CAD build for the part. Positions are in the model's coordinates, mm. A direction names the side the tool comes from. Round coordinates to 2 decimals unless told otherwise and drop trailing zeros. Order: outer loops, then holes, each group sorted by start corner. A loop starts at its lowest first (then second) coordinate and runs counter-clockwise, first axis right, second up. Notation, with made-up numbers: (-21, 52.25) - (8, 52.25) arc R26 cw to (8, 69.25) - close; hole circle Ø10 at (74.25, -20). An arc over 180 degrees is marked (long way). Use one line per item in the form item = value. Start each with the question number.
Autodesk Inventor part; units mm, degrees
ref_plane "Work Plane1" through (443.7901, 0, 457.2) normal (-0.7071, 0, 0.7071) x (0, -1, 0)
ref_plane "YZ Plane" through (0, 0, 0) normal (1, 0, 0) x (0, 1, 0)
ref_plane "XZ Plane" through (0, 0, 0) normal (0, 1, 0) x (-1, 0, 0)
sketch "Sketch1" plane through (0, 0, 0) normal (0, 0, 1) x (1, 0, 0)
  line L0 (-13.4099, 13.8043) -> (443.7901, 13.8043)
  line L1 (443.7901, 13.8043) -> (443.7901, -443.3957)
  line L2 (443.7901, -443.3957) -> (-13.4099, -443.3957)
  line L3 (-13.4099, -443.3957) -> (-13.4099, 13.8043)
  point P0 (0, 0)
  dimension "d0" = 457.2
  dimension "d1" = 457.2
extrude "Extrusion1" add sketch "Sketch1" along normal blind 457.2
ref_plane "Work Plane1" through (443.7901, 0, 457.2) normal (-0.7071, 0, 0.7071) x (0, -1, 0)
sketch "Sketch2" plane through (0, 0, 457.2) normal (0, 0, 1) x (1, 0, 0)
  point P0 (0, 0)
sketch "Sketch3" plane through (0, 0, 457.2) normal (0, 0, 1) x (1, 0, 0)
  circle A0 centre (215.1901, -214.7957) radius 78.8174
  line L0 (443.7901, -443.3957) -> (443.7901, 13.8043)
  line L1 (443.7901, 13.8043) -> (-13.4099, 13.8043)
  point P0 (0, 0)
  dimension "d4" = 228.6
  dimension "d5" = 228.6
extrude "Extrusion2" add sketch "Sketch3" along normal blind 12.7
sketch "Sketch4" plane through (443.7901, -443.3957, 0) normal (1, 0, 0) x (0, 0, -1)
  point P0 (0, 443.3957)
sketch "Sketch5" plane through (443.7901, -443.3957, 0) normal (1, 0, 0) x (0, 0, -1)
  line L0 (0, 457.2) -> (-457.2, 0)
  circle A0 centre (-76.1993, 381.0007) radius 63.5
  circle A1 centre (-228.6, 228.6) radius 63.5
  circle A2 centre (-381.0007, 76.1993) radius 63.5
  point P0 (0, 443.3957)
  dimension "d21" = 127
  dimension "d22" = 127
  dimension "d23" = 127
  dimension "d25" = 646.5784
  dimension "d26" = 107.762
  dimension "d28" = 107.762
extrude "Extrusion3" add sketch "Sketch5" along normal blind 12.7
sketch "Sketch6" plane through (-13.4099, -443.3957, 0) normal (-1, 0, 0) x (0, 0, 1)
  line L0 (0, 457.2) -> (457.2, 0)
  line L1 (114.3, 342.9) -> (342.9, 342.9)
  line L2 (342.9, 342.9) -> (342.9, 114.3)
  line L3 (342.9, 114.3) -> (114.3, 114.3)
  line L4 (114.3, 114.3) -> (114.3, 342.9)
  line L5 (0, 0) -> (0, 457.2)
  line L6 (457.2, 457.2) -> (457.2, 0)
  circle A0 centre (114.3, 342.9) radius 63.5
  circle A1 centre (342.9, 342.9) radius 63.5
  circle A2 centre (114.3, 114.3) radius 63.5
  circle A3 centre (342.9, 114.3) radius 63.5
  point P0 (228.6, 228.6)
  dimension "d37" = 228.6
  dimension "d38" = 114.3
  dimension "d40" = 127
  dimension "d41" = 127
  dimension "d42" = 127
  dimension "d43" = 127
extrude "Extrusion4" add sketch "Sketch6" along normal blind 12.7 contours A0 L1 L0 | L0 L4 A0 | L1 A0 L0 | L0 A0 L4 | A1 L2 L1 | L1 L2 A1 | A2 L3 L4 | L4 L3 A2 | A3 L2 L0 | L0 L3 A3 | L2 A3 L0 | L0 A3 L3
sketch "Sketch7" plane through (0, 0, 0) normal (0, 0, -1) x (-1, 0, 0)
  line L0 (-443.7901, 13.8043) -> (-316.7901, 13.8043)
  line L1 (-443.7901, 13.8043) -> (13.4099, 13.8043)
  line L2 (13.4099, 13.8043) -> (-113.5901, 13.8043)
  line L3 (-443.7901, -443.3957) -> (13.4099, -443.3957)
  line L4 (-316.7901, 13.8043) -> (-316.7901, -443.3957)
  line L5 (-113.5901, 13.8043) -> (-113.5901, -443.3957)
  line L6 (-316.7901, 13.8043) -> (-316.7901, -62.3957)
  line L7 (-316.7901, -443.3957) -> (-316.7901, -367.1957)
  circle A0 centre (-316.7901, -62.3957) radius 63.5
  circle A1 centre (-316.7901, -367.1957) radius 63.5
  circle A2 centre (-316.7901, -214.7957) radius 63.5
  circle A3 centre (-113.5901, -62.3957) radius 63.5
  circle A4 centre (-113.5901, -214.7957) radius 63.5
  circle A5 centre (-113.5901, -367.1957) radius 63.5
  point P0 (0, 0)
  dimension "d46" = 127
  dimension "d47" = 127
  dimension "d53" = 76.2
  dimension "d54" = 76.2
  dimension "d55" = 127
  dimension "d56" = 127
  dimension "d57" = 127
  dimension "d58" = 127
  dimension "d59" = 127
  dimension "d60" = 127
extrude "Extrusion5" add sketch "Sketch7" along normal blind 12.7 contours A0 L4 | L4 A0 | A3 L5 | L5 A3 | A2 L4 | L4 A2 | A4 L5 | L5 A4 | A1 L4 | L4 A1 | A5 L5 | L5 A5
sketch "Sketch8" plane through (-13.4099, 13.8043, 0) normal (0, 1, 0) x (1, 0, 0)
  line L0 (355.6, -101.6) -> (101.6, -101.6)
  line L1 (101.6, -101.6) -> (101.6, -355.6)
  line L2 (101.6, -355.6) -> (355.6, -355.6)
  line L3 (355.6, -355.6) -> (355.6, -101.6)
  line L4 (355.6, -101.6) -> (101.6, -355.6)
  circle A0 centre (355.6, -101.6) radius 63.5
  line L5 (0, 0) -> (457.2, 0)
  line L6 (457.2, -457.2) -> (0, -457.2)
  line L7 (457.2, 0) -> (457.2, -457.2)
  circle A1 centre (228.6, -228.6) radius 63.5
  circle A2 centre (101.6, -101.6) radius 63.5
  circle A3 centre (101.6, -355.6) radius 63.5
  circle A4 centre (355.6, -355.6) radius 63.5
  point P0 (13.4099, 0)
  dimension "d63" = 254
  dimension "d64" = 101.6
  dimension "d65" = 101.6
  dimension "d66" = 101.6
  dimension "d67" = 127
  dimension "d68" = 127
  dimension "d69" = 127
  dimension "d70" = 127
  dimension "d71" = 127
extrude "Extrusion6" add sketch "Sketch8" along normal blind 12.7 contours A2 L1 L0 | L0 L1 A2 | A0 L3 L0 | L0 L4 A0 | L3 A0 L4 | A3 L4 L1 | L1 L2 A3 | A1 L4 | L4 A1 | L4 A3 L2 | A4 L2 L3 | L3 L2 A4
sketch "Sketch9" plane through (-13.4099, -443.3957, 0) normal (0, -1, 0) x (1, 0, 0)
  line L0 (0, 0) -> (457.2, 457.2)
  line L1 (457.2, 457.2) -> (304.8, 304.8)
  line L2 (0, 0) -> (152.4, 152.4)
  circle A0 centre (152.4, 152.4) radius 63.5
  circle A1 centre (304.8, 304.8) radius 63.5
  point P0 (13.4099, 0)
  dimension "d77" = 646.5784
  dimension "d78" = 127
  dimension "d79" = 127
extrude "Extrusion7" add sketch "Sketch9" along normal blind 12.7
properties part number "dicemodel1"
(1) Which spindle directions (+Z, -Z, +X, -X, +Y, -Y) get a long thin tool onto all of the face, cutting with end or side? Do faces 4 (the cylindrical face through (75.55, -449.66, 149.61)), 5 (the cylindrical face through (367.182, -176.157, -6.261)), 6 (the cylindrical face through (402.76, 20.07, 120.67)), 7 (the flat face through (443.79, -262, 175)), 8 (the cylindrical face through (-19.671, -392.055, 106.034)). Say none if no direction does.
(2) Slice it at D-D (x = 387.5). Give the cut face in (y, z).
(3) Mould opens along Y. For faces 1 (the cylindrical face through (450.051, -190.475, 169.942)), 2 (the cylindrical face through (244.491, 20.065, 172.265)), 3 (the cylindrical face through (84.29, -158.46, -6.26)) say: pulls with the +Y half, pulls with the -Y half, needs draft (parallel to the pull), parting line crosses it, or undercut.
(4) Flat gauge pins, fed straight in: P1, Ø1.5, axis at y = -260.5, z = 381, coming from the +X side; P2, Ø10, axis at x = 122.5, y = -321.5, coming from the +Z side; P3, Ø1, axis at x = 148.5, z = 410, coming from the +Y side. Where does each tip first touch, or does it go through?
(5) Slice it at A-A (z = 228.6). Give the cut face in (x, y).
(6) Wall check: line 1 (X direction, y = -276.5, z = 265); line 2 (Z direction, x = 355.5, y = -303); line 3 (Z direction, x = 352.5, y = -389). Give the ranges that are in metal, low to high. Write a range as [from, to].
(7) Slice it at B-B (x = 60.5). Give the cut face in (y, z).
(8) Slice it at C-C (y = -385.5). Give the cut face in (x, z), and give its area (3 significant figures).
Results list:
q1.face_4 = -Y
q1.face_5 = -Z
q1.face_6 = +Y
q1.face_7 = +X
q1.face_8 = -X
q2.outline = (-443.4, 0) - (13.8, 0) - (13.8, 57.11) - (26.5, 57.11) - (26.5, 146.09) - (13.8, 146.09) - (13.8, 311.11) - (26.5, 311.11) - (26.5, 400.09) - (13.8, 400.09) - (13.8, 457.2) - (-443.4, 457.2) - close
q3.face_1 = parting line crosses it
q3.face_2 = needs draft
q3.face_3 = undercut
q4.P1 = 443.79
q4.P2 = 457.2
q4.P3 = 13.8
q5.outline = (-13.41, -443.4) - (443.79, -443.4) - (443.79, -278.3) - (456.49, -278.3) - (456.49, -151.3) - (443.79, -151.3) - (443.79, 13.8) - (278.69, 13.8) - (278.69, 26.5) - (151.69, 26.5) - (151.69, 13.8) - (-13.41, 13.8) - close
q6.line_1 = [-13.41, 443.79]
q6.line_2 = [0, 457.2]
q6.line_3 = [-12.7, 457.2]
q7.outline = (-443.4, 0) - (-402.03, 0) - (-402.03, -12.7) - (-332.36, -12.7) - (-332.36, 0) - (-249.63, 0) - (-249.63, -12.7) - (-179.96, -12.7) - (-179.96, 0) - (-97.23, 0) - (-97.23, -12.7) - (-27.56, -12.7) - (-27.56, 0) - (13.8, 0) - (13.8, 44.46) - (26.5, 44.46) - (26.5, 158.74) - (13.8, 158.74) - (13.8, 298.46) - (26.5, 298.46) - (26.5, 412.74) - (13.8, 412.74) - (13.8, 457.2) - (-443.4, 457.2) - close
q8.outline = (-26.11, 85.13) - (-13.41, 85.13) - (-13.41, 0) - (52.79, 0) - (52.79, -12.7) - (174.39, -12.7) - (174.39, 0) - (255.99, 0) - (255.99, -12.7) - (377.59, -12.7) - (377.59, 0) - (443.79, 0) - (443.79, 320.2) - (456.49, 320.2) - (456.49, 441.81) - (443.79, 441.81) - (443.79, 457.2) - (-13.41, 457.2) - (-13.41, 372.07) - (-26.11, 372.07) - (-26.11, 313.73) - (-13.41, 313.73) - (-13.41, 143.47) - (-26.11, 143.47) - close
q8.area = 215,000 mm²
